Could you check a few things on this drawing? It's one solid part, dimensions in mm from its lowest x, y, z. A direction names the side the tool comes from. Round coordinates to 2 decimals unless told otherwise and drop trailing zeros. Write each loop counter-clockwise with the first axis right and the second up, starting at its lowest first coordinate (ties: lowest second). Pieces come first, ordered by that corner, then holes. Notation, with made-up numbers: (18, -35.75) - (61, -35.75) arc R14 cw to (61, -28.75) - close; hole circle Ø10 at (16, -32). An arc over 180 degrees is marked (long way). One line per question, with ' | ' between items. Start each with the question number.
(1) Will these pins go through, and if not, where does the flat tip stop? pin 1 (2.5 mm diameter, centred on x = 8.5, z = 11.5, fed in from +Y); pin 2 (5 mm diameter, centred on x = 30.5, z = 10, fed in from +Y); pin 3 (4 mm diameter, centred on x = 25.5, z = 8, fed in from +Y).
(2) Imagine slicing it at B-B (x = 8.5). Write out the boundary of the cut face in (y, z), plus the area to 3 significant figures.
(3) Imagine slicing it at A-A (y = 8.75). Write out the boundary of the cut face in (x, z), plus the area to 3 significant figures.
(4) Imagine slicing it at C-C (z = 9.25). Write out the boundary of the cut face in (x, y).
(5) Imagine slicing it at D-D (x = 28.5). Write out the boundary of the cut face in (y, z).
(6) For the marked faces 5 and 6, which set-ups out of +Z, -Z, +X, -X, +Y, -Y let a thin tool reach every point of the face, with its end or its side?
(7) Thinking about a two-plate mould opening in X: for the marked faces 1, 2, 3 and 4, which applies, pulls with the +X half, pulls with the -X half, needs draft (parallel to the pull), parting line crosses it, or undercut?
(8) If I drill on L1, parallel to X at y = 3.5, z = 8.5; L2, parallel to Z at x = 11, y = 9.5; L3, parallel to X at y = 2.5, z = 11, over which ranges is the centre line in solid material (lowest first)?
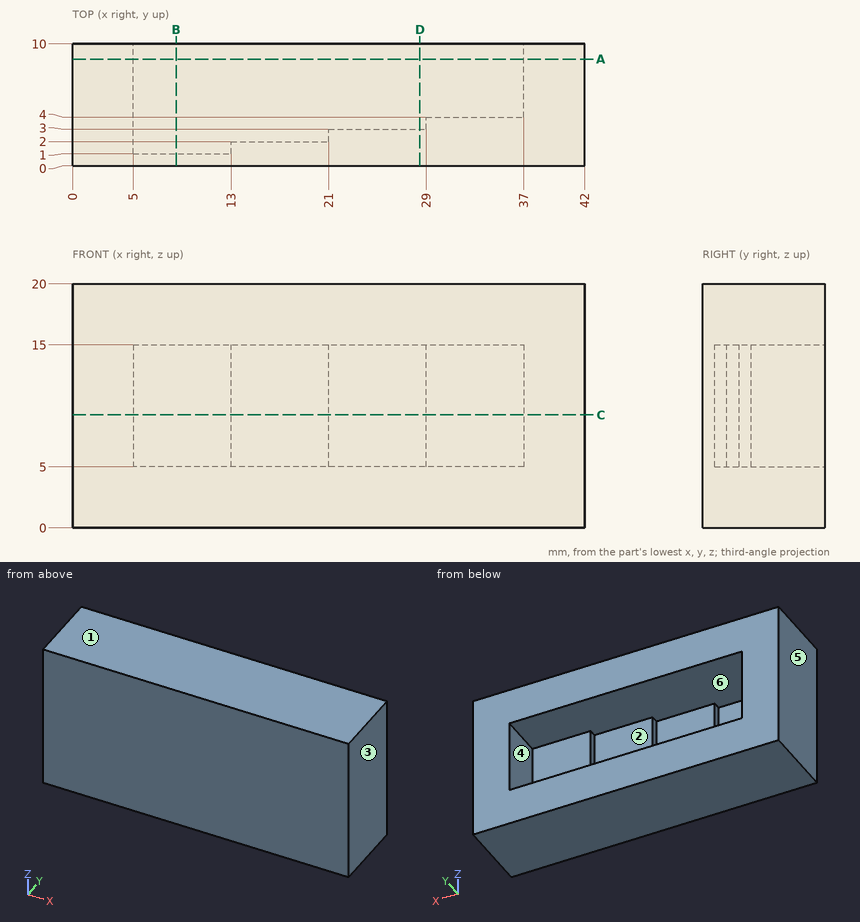
Check sheet entries:
1) pin 1: y = 1 | pin 2: y = 4 | pin 3: y = 3
2) outline: (0, 0) - (10, 0) - (10, 5) - (1, 5) - (1, 15) - (10, 15) - (10, 20) - (0, 20) - close | area: 110 mm^2
3) outline: (0, 0) - (42, 0) - (42, 20) - (0, 20) - close; hole (5, 5) - (37, 5) - (37, 15) - (5, 15) - close | area: 520 mm^2
4) outline: (0, 0) - (42, 0) - (42, 10) - (37, 10) - (37, 4) - (29, 4) - (29, 3) - (21, 3) - (21, 2) - (13, 2) - (13, 1) - (5, 1) - (5, 10) - (0, 10) - close
5) outline: (0, 0) - (10, 0) - (10, 5) - (3, 5) - (3, 15) - (10, 15) - (10, 20) - (0, 20) - close
6) face 5: +Z, -Z, -X, +Y, -Y | face 6: +Y
7) face 1: needs draft | face 2: undercut | face 3: pulls with the +X half | face 4: undercut
8) L1: 0 to 5, 29 to 42 | L2: 0 to 5, 15 to 20 | L3: 0 to 5, 21 to 42
